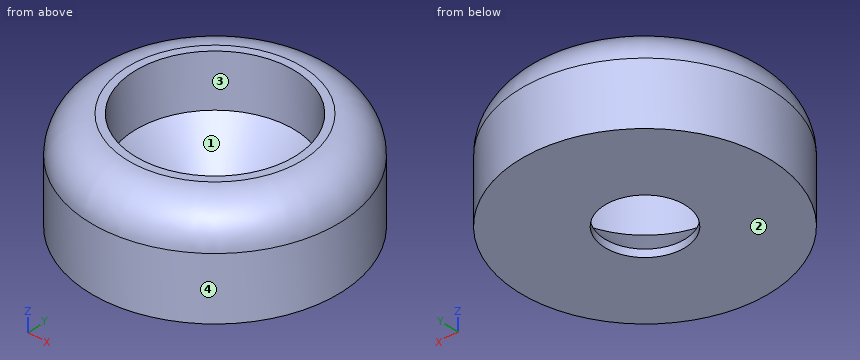
from build123d import *

# Parameters (mm, degrees)
SKETCH1_R           = 5
SKETCH1_R_2         = 1.6
BOSS_EXTRUDE1_DEPTH = 4
SKETCH2_R           = 3.2
CUT_EXTRUDE1_DEPTH  = 1.9
CHAMFER1_SIZE       = 1.8
FILLET1_R           = 1.5


with BuildPart() as part:
    # Sketch1 → Boss-Extrude1 (new body)
    with BuildSketch(Plane.XY):
        Circle(SKETCH1_R)
        Circle(SKETCH1_R_2, mode=Mode.SUBTRACT)
    extrude(amount=BOSS_EXTRUDE1_DEPTH)

    # Sketch2 → Cut-Extrude1 (cut)
    with BuildSketch(Plane.XY.offset(4)):
        Circle(SKETCH2_R)
    extrude(amount=-CUT_EXTRUDE1_DEPTH, mode=Mode.SUBTRACT)

    # Chamfer1
    # the kernel refuses this chamfer: 1.8 mm, written as the material it takes off along each edge
    with BuildSketch(Plane(origin=(0, 0, 2.1), x_dir=(1, 0, 0), z_dir=(0, 1, 0))) as chamfer1_piece_1_section:
        Polygon((1.6, CHAMFER1_SIZE), (1.6 + CHAMFER1_SIZE, 0), (1.6, 0), align=None)
    chamfer1_piece_1 = revolve(axis=Axis((0, 0, 2.1), (0, 0, -1)), mode=Mode.PRIVATE)
    chamfer1_piece_1 = chamfer1_piece_1 & Plane(origin=(0, 0, 1.094879123), x_dir=(1, 0, 0), z_dir=(0, 0, 1)) * Cylinder(3.2, 14, mode=Mode.PRIVATE)
    add(chamfer1_piece_1, mode=Mode.SUBTRACT)

    # Fillet1
    fillet1_edges = [part.edges().sort_by_distance(p)[0] for p in [
        (-5, 0, 4),
    ]]
    fillet(fillet1_edges, radius=FILLET1_R)


solid = part.part
Design review of the part built by this model. Coordinates are the model's own, in mm. Face numbers are marked on the shaded views. Coordinates: 2 decimals unless noted, no trailing zeros. Order: outer loops, then holes, each group sorted by start corner. A loop starts at its lowest first (then second) coordinate and runs counter-clockwise, first axis right, second up. Notation, with made-up numbers: (13, 7) -> (61, 7) arc R29 cw to (61, 45) -> close; hole circle Ø7 at (-8.75, 77.5). An arc over 180 degrees is marked (long way). Use one line per item in the form item = value. Start each with the question number.
(1) Add section B-B on z = 1.3. State the section outline as (x, y) points, plus the area to 3 significant figures.
(2) Insertion check: pin 1 (4 mm diameter, centred on x = 3, y = -1.5, fed in from -Z). The pin has a flat end and moves straight along its axis. Give the tip position at first contact, or say it passes through.
(3) Add section A-A on x = 0. State the section outline as (y, z) points.
(4) For probe 1 along Y at (x, z) = (0, 0.2); probe 2 along Y at (x, z) = (2.5, 2.7); probe 3 along Z at (x, y) = (-2, -0.5), list the stretches that pass through material, from the lowest coordinate up.
(5) The part is to be moulded in two halves that separate along Y. For the marked faces 1, 2, 3 and 4, say which applies: +Y half, -Y half, draft (parallel to the pull), parting line (faces both ways), or undercut.
Answer block:
q1.outline = circle Ø10 at (0, 0); hole circle Ø5.2 at (0, 0)
q1.area = 57.3 mm²
q2.pin_1 = 0
q3.outline = (-5, 0) -> (-1.6, 0) -> (-1.6, 0.3) -> (-3.2, 1.9) -> (-3.2, 4) -> (-3.5, 4) arc R1.5 ccw to (-5, 2.5) -> close; (1.6, 0) -> (5, 0) -> (5, 2.5) arc R1.5 ccw to (3.5, 4) -> (3.2, 4) -> (3.2, 1.9) -> (1.6, 0.3) -> close
q4.probe_1 = -5 to -1.6, 1.6 to 5
q4.probe_2 = -4.31 to -2, 2 to 4.31
q4.probe_3 = 0 to 0.76
q5.face_1 = undercut
q5.face_2 = draft
q5.face_3 = undercut
q5.face_4 = parting line
